```python
from build123d import *

# Parameters (mm, degrees)
SKETCH1_W           = 110
SKETCH1_H           = 164
BOSS_EXTRUDE1_DEPTH = 2.9
SKETCH2_W           = 110
SKETCH2_H           = 2
REVOLVE1_ANGLE      = 180


with BuildPart() as part:
    # Sketch1 → Boss-Extrude1 (new body)
    with BuildSketch(Plane(origin=(0, 0, 0), x_dir=(1, 0, 0), z_dir=(0, 1, 0))):
        with Locations((55, -82)):
            Rectangle(SKETCH1_W, SKETCH1_H)
    extrude(amount=BOSS_EXTRUDE1_DEPTH)

    # Sketch2 → Revolve1 (revolve)
    with BuildSketch(Plane(origin=(0, 2.9, 0), x_dir=(1, 0, 0), z_dir=(0, 1, 0))):
        with Locations((55, -163)):
            Rectangle(SKETCH2_W, SKETCH2_H)
    revolve(axis=Axis((110, 2.9, 162), (-1, 0, 0)), revolution_arc=REVOLVE1_ANGLE)


solid = part.part
```
The model under review builds one solid part; all positions refer to its coordinate system, in mm. A direction names the side the tool comes from. Coordinates: 2 decimals unless noted, no trailing zeros. Write each loop counter-clockwise with the first axis right and the second up, starting at its lowest first coordinate (ties: lowest second). Pieces come first, ordered by that corner, then holes. Notation, with made-up numbers: (77, 39.5) - (127, 39.5) arc R26 ccw to (127, 72.5) - close; hole circle Ø9 at (31, 72.5). An arc over 180 degrees is marked (long way). Write item = value, one per line.
(1) For P1, Ø5, axis at x = 19, z = 34.5, coming from the -Y side; P2, Ø2, axis at x = 12, z = 85, coming from the +Y side, all flat-tipped, find the tip position at first contact; note any pin that passes through.
Result sheet:
P1 = 0
P2 = 2.9
(2) Machinability: for faces 1 (the face through (54, 2.9, 79)), 2 (the face through (54, 0, 81)), which of the approach directions +Z, -Z, +X, -X, +Y, -Y give a long, thin tool a straight path to every point of the face, cutting with its end or side? Answer none if there is none.
Result sheet:
face_1 = -Z, +X, -X, +Y
face_2 = +Z, -Z, +X, -X, -Y
(3) For line 1 (Y direction, x = 47, z = 77); line 2 (Z direction, x = 97, y = 4.6); line 3 (Z direction, x = 93, y = 4.2), list the stretches that pass through material, from the lowest coordinate up. Write a range as [from, to].
Result sheet:
line_1 = [0, 2.9]
line_2 = [160.95, 163.05]
line_3 = [160.48, 163.52]
(4) Consider section B-B, the plane z = 147. Give the boundary of the cut face in (x, y).
Result sheet:
outline = (0, 0) - (110, 0) - (110, 2.9) - (0, 2.9) - close
(5) Consider section A-A, the plane x = 78. Give the boundary of the cut face in (y, z).
Result sheet:
outline = (0, 0) - (2.9, 0) - (2.9, 160) arc R2 ccw to (2.9, 164) - (0, 164) - close
